from build123d import *

# Parameters (mm, degrees)
BOSS_EXTRUDE1_DEPTH = 10
M3_TAPPED_HOLE1_D   = 3
FILLET1_R           = 0.1


with BuildPart() as part:
    # Sketch1 → Boss-Extrude1 (new body)
    with BuildSketch(Plane.XY):
        Polygon((1.508379031, 2.461326072), (-1.37738139, 2.536957595), (-2.885760421, 0.075631523), (-1.508379031, -2.461326072), (1.37738139, -2.536957595), (2.885760421, -0.075631523), align=None)
    extrude(amount=BOSS_EXTRUDE1_DEPTH)

    # M3 Tapped Hole1 (through all)
    with Locations(Plane.XY.offset(10)):
        with Locations((0, 0)):
            Hole(M3_TAPPED_HOLE1_D / 2)

    # Fillet1
    fillet1_edges = [part.edges().sort_by_distance(p)[0] for p in [
        (2.885760421, -0.075631523, 5),
        (1.37738139, -2.536957595, 5),
        (-1.508379031, -2.461326072, 5),
        (-2.885760421, 0.075631523, 5),
        (-1.37738139, 2.536957595, 5),
        (1.508379031, 2.461326072, 5),
    ]]
    fillet(fillet1_edges, radius=FILLET1_R)


solid = part.part
The model under review builds one solid part; all positions refer to its coordinate system, in mm. Give positions to 0.01 mm unless a question says otherwise; leave off trailing zeros. Order: outer loops, then holes, each group sorted by start corner. A loop starts at its lowest first (then second) coordinate and runs counter-clockwise, first axis right, second up. Notation, with made-up numbers: M 66,-4 L 99,-4 A18 ccw 99,3 Z; hole C 1,50.5 d1. An arc over 180 degrees is marked long. Use one line per item in the form item = value. Start each with the question number.
Item 1: The part is to be moulded in two halves that separate along X. For faces 1 (the flat face through (2.206, 1.176, 4.93)), 2 (the cylindrical face through (1.5, 0.07, 4.93)), 3 (the flat face through (1.2, 1.2, 0)), say which applies: pulls with the +X half, pulls with the -X half, needs draft (parallel to the pull), parting line crosses it, or undercut.
Item 2: Insertion check: pin 1 Ø1.8 at (x, y) = (0, 0) entering from +Z. The pin has a flat end and moves straight along its axis. Give the tip position at first contact, or say it passes through.
Item 3: We need section A-A on z = 3.5. Give the boundary of the cut face in (x, y).
Item 4: We need section C-C on y = -1.75. Give the boundary of the cut face in (x, z).
Item 5: We need section B-B on x = -0.45. Give the boundary of the cut face in (y, z).
Item 6: To check wall thickness, follow line 1 along Y through (x, z) = (0, 2.5); line 2 along X through (y, z) = (1.3, 4.25); line 3 along Y through (x, z) = (-0.75, 2). State the ranges of each line that lie inside material, in increasing order. Write a range as from..to.
Item 7: We need section D-D on x = 2.05. Give the boundary of the cut face in (y, z).
Completed:
q1.face_1 = pulls with the +X half
q1.face_2 = undercut
q1.face_3 = needs draft
q2.pin_1 = through
q3.outline = M -2.86,0.02 L -1.54,-2.41 A0.1 ccw -1.45,-2.46 L 1.32,-2.54 A0.1 ccw 1.41,-2.49 L 2.86,-0.12 A0.1 ccw 2.86,-0.02 L 1.54,2.41 A0.1 ccw 1.45,2.46 L -1.32,2.54 A0.1 ccw -1.41,2.49 L -2.86,0.12 A0.1 ccw Z; hole C 0,0 d3
q4.outline = M -1.89,0 L 1.86,0 L 1.86,10 L -1.89,10 Z
q5.outline = M -2.49,0 L -1.43,0 L -1.43,10 L -2.49,10 Z; M 1.43,0 L 2.51,0 L 2.51,10 L 1.43,10 Z
q6.line_1 = -2.5..-1.5, 1.5..2.5
q6.line_2 = -2.14..-0.75, 0.75..2.14
q6.line_3 = -2.48..-1.3, 1.3..2.52
q7.outline = M -1.44,0 L 1.46,0 L 1.46,10 L -1.44,10 Z
